Part model, mm, in its own coordinate system. Face numbers are marked on the shaded views. A direction names the side the tool comes from. Give positions to 0.01 mm unless a question says otherwise; leave off trailing zeros. Order: outer loops, then holes, each group sorted by start corner. A loop starts at its lowest first (then second) coordinate and runs counter-clockwise, first axis right, second up. Notation, with made-up numbers: M 31,30.5 L 64,30.5 A27 cw 64,59.5 Z; hole C 70.25,36 d4. An arc over 180 degrees is marked long. Return JSON: item names as keys, results as strings.
from build123d import *

# Parameters (mm, degrees)
SKETCH_W     = 25.4
SKETCH_H     = 25.4
SKETCH_R     = 3.3782
PAD_DEPTH    = 2
SKETCH001_W  = 25.4
SKETCH001_H  = 25.4
SKETCH001_R  = 3.3782
PAD001_DEPTH = 2
PAD002_DEPTH = 2


with BuildPart() as part:
    # Sketch → Pad (new body)
    with BuildSketch(Plane.XY):
        with Locations((0, 12.7)):
            Rectangle(SKETCH_W, SKETCH_H)
        with Locations((0, 12.7)):
            Circle(SKETCH_R, mode=Mode.SUBTRACT)
    extrude(amount=PAD_DEPTH)

    # Sketch001 → Pad001 (join)
    with BuildSketch(Plane.XZ):
        with Locations((0, -12.7)):
            Rectangle(SKETCH001_W, SKETCH001_H)
        with Locations((0, -12.7)):
            Circle(SKETCH001_R, mode=Mode.SUBTRACT)
    extrude(amount=-PAD001_DEPTH)

    # Sketch002 (on Face9 of Pad001) → Pad002 (join)
    with BuildSketch(Plane.YZ.offset(12.7)):
        Polygon((2, -25.4), (2, 0), (25.4, 0), align=None)
    pad002 = extrude(amount=-PAD002_DEPTH)

    # Mirrored: Pad002 across YZ
    add(pad002.mirror(Plane.YZ))


solid = part.part
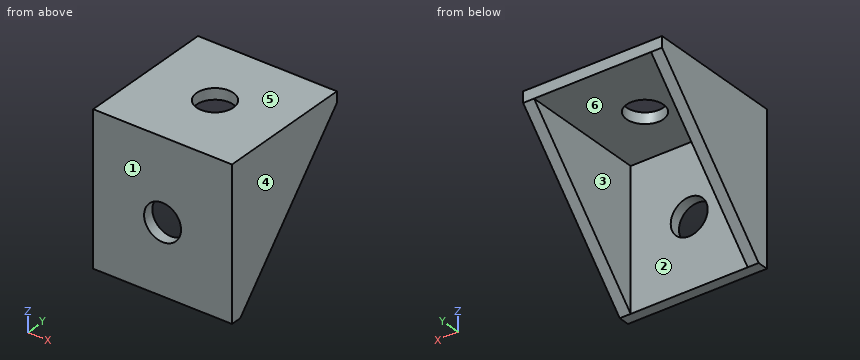
Q1. Two-plate mould, pull along X, no slides. Class the marked faces 3, 4, 5 and 6: +X half, -X half, draft (parallel to the pull), parting line (faces both ways), or undercut.
Established:
{"face 3": "undercut", "face 4": "+X half", "face 5": "draft", "face 6": "undercut"}
Q2. Band-saw the part on A-A (z = -12.7). Give the cut face in (x, y), then the cut area to 3 significant figures.
Established:
{"outline": "M -12.7,0 L -3.38,0 L -3.38,2 L -10.7,2 L -10.7,13.7 L -12.7,13.7 Z; M 3.38,0 L 12.7,0 L 12.7,13.7 L 10.7,13.7 L 10.7,2 L 3.38,2 Z", "area": "84.1 mm²"}
Q3. Pin check, flat tips, straight feed: pin 1 (11 mm diameter, centred on x = 0, y = 12.7, fed in from -Z); pin 2 (8 mm diameter, centred on x = 8, y = 21.5, fed in from -Z); pin 3 (10.5 mm diameter, centred on x = -4, z = -15.5, fed in from +Y). Stop position of each tip, or through.
Established:
{"pin 1": "stops at z = 0", "pin 2": "stops at z = -7.44", "pin 3": "stops at y = 2"}
Q4. 3-axis set-ups, long thin cutter, end or side, ignore diameter. For the marked faces 1 and 2: which of +Z, -Z, +X, -X, +Y, -Y reach the whole face in a straight line?
Established:
{"face 1": "+Z, -Z, +X, -X, -Y", "face 2": "-Z, +Y"}
Q5. Band-saw the part on C-C (y = 12.7). Give the cut face in (x, z), then the cut area to 3 significant figures.
Established:
{"outline": "M -12.7,-13.79 L -10.7,-13.79 L -10.7,0 L -3.38,0 L -3.38,2 L -12.7,2 Z; M 3.38,0 L 10.7,0 L 10.7,-13.79 L 12.7,-13.79 L 12.7,2 L 3.38,2 Z", "area": "92.4 mm²"}
Q6. Probe line 1 along X through (y, z) = (8, -3); line 2 along Y through (x, z) = (0, 0.4); line 3 along Z through (x, y) = (0, 1.1). List the from-to ranges inside material, lowest first.
Established:
{"line 1": "x = -12.7 to -10.7, 10.7 to 12.7", "line 2": "y = 0 to 9.32, 16.08 to 25.4", "line 3": "z = -25.4 to -16.08, -9.32 to 2"}
Q7. Band-saw the part on D-D (z = -1). Give the cut face in (x, y).
Established:
{"outline": "M -12.7,0 L 12.7,0 L 12.7,24.48 L 10.7,24.48 L 10.7,2 L -10.7,2 L -10.7,24.48 L -12.7,24.48 Z"}
Q8. Band-saw the part on B-B (x = 0). Give the cut face in (y, z), then the cut area to 3 significant figures.
Established:
{"outline": "M 0,-25.4 L 2,-25.4 L 2,-16.08 L 0,-16.08 Z; M 0,-9.32 L 2,-9.32 L 2,0 L 9.32,0 L 9.32,2 L 0,2 Z; M 16.08,0 L 25.4,0 L 25.4,2 L 16.08,2 Z", "area": "74.6 mm²"}
